from build123d import *

# Parameters (mm, degrees)
SKETCH1_W           = 35
SKETCH1_H           = 35
BOSS_EXTRUDE1_DEPTH = 3
SKETCH2_R           = 10
BOSS_EXTRUDE2_DEPTH = 5


with BuildPart() as part:
    # Sketch1 → Boss-Extrude1 (new body)
    with BuildSketch(Plane(origin=(0, 0, 0), x_dir=(1, 0, 0), z_dir=(0, 1, 0))):
        with Locations((17.5, -17.5)):
            Rectangle(SKETCH1_W, SKETCH1_H)
    extrude(amount=-BOSS_EXTRUDE1_DEPTH)

    # Sketch2 → Boss-Extrude2 (add)
    with BuildSketch(Plane(origin=(0, 0, 0), x_dir=(1, 0, 0), z_dir=(0, 1, 0))):
        with Locations(Location((17.5, -10.9375, 0), (0, 0, 270))):
            Circle(SKETCH2_R)
    extrude(amount=BOSS_EXTRUDE2_DEPTH)


solid = part.part
Work out the finished part from the listing and answer in its coordinate system (mm). Coordinates: 2 decimals unless noted, no trailing zeros. Write each loop counter-clockwise with the first axis right and the second up, starting at its lowest first coordinate (ties: lowest second). Pieces come first, ordered by that corner, then holes. Notation, with made-up numbers: M 61.5,12.5 L 85.5,12.5 A11 ccw 85.5,22.5 Z; hole C 79,85 d4. An arc over 180 degrees is marked long. Use one line per item in the form item = value. Start each with the question number.
1. The part is cut by section C-C (y = 1.25). Give the vertices of the cut face in (x, z).
2. The part is cut by section B-B (z = 11). Give the vertices of the cut face in (x, y).
3. The part is cut by section D-D (x = 2.5). Give the vertices of the cut face in (y, z), plus the area to 3 significant figures.
4. Straight lines are drawn through the part: probe 1 along X at (y, z) = (1.75, 11); probe 2 along Y at (x, z) = (3, 16); probe 3 along Z at (x, y) = (18.5, 2). For each, find the intervals that lie inside material, in ascending order. Write a range as from..to.
5. Each of these flat-tipped pins is pushed along its axis until it touches: P1, Ø2, axis at y = 0, z = 15.5, coming from the -X side; P2, Ø1.5, axis at x = 7.5, y = 1.5, coming from the -Z side; P3, Ø3, axis at y = 3.5, z = 17, coming from the +X side. Where does it stop, or does it pass through?
6. The mould has two halves that part along X. Classify faces 1 (the face through (35, -1, 18)), 2 (the face through (17, -1, 35)), 3 (the face through (24.26, 2.46, 3.57)), 4 (the face through (0, -1, 18)): released by +X, released by -X, zero draft, split by the parting line, or undercut.
7. The part is cut by section A-A (x = 17.5). Give the vertices of the cut face in (y, z).
Evaluation:
q1.outline = C 17.5,10.94 d20
q2.outline = M 0,-3 L 35,-3 L 35,0 L 27.5,0 L 27.5,5 L 7.5,5 L 7.5,0 L 0,0 Z
q3.outline = M -3,0 L 0,0 L 0,35 L -3,35 Z
q3.area = 105 mm^2
q4.probe_1 = 7.5..27.5
q4.probe_2 = -3..0
q4.probe_3 = 0.99..20.89
q5.P1 = 0
q5.P2 = 7.14
q5.P3 = 26.4
q6.face_1 = released by +X
q6.face_2 = zero draft
q6.face_3 = split by the parting line
q6.face_4 = released by -X
q7.outline = M -3,0 L 0,0 L 0,0.94 L 5,0.94 L 5,20.94 L 0,20.94 L 0,35 L -3,35 Z
